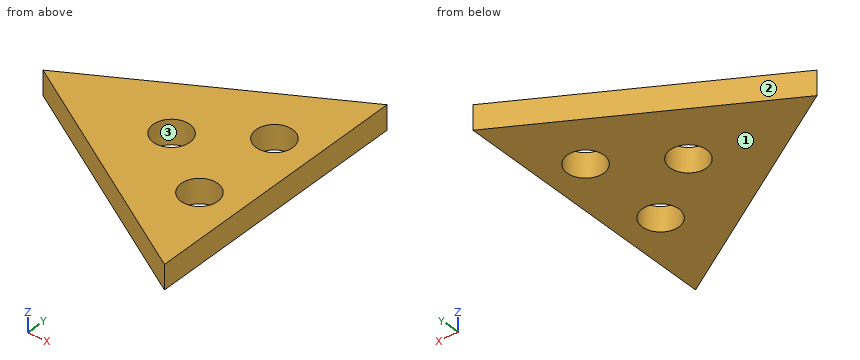
```python
from build123d import *

# Parameters (mm, degrees)
F0_R     = 1.5
F1_DEPTH = 2


with BuildPart() as f1:
    # F0 (on Top) → F1 (new body)
    with BuildSketch(Plane.XY):
        Polygon((9.526279, 11), (-9.526279, 0), (9.526279, -11), (9.526279, -10), (9.526279, 10), align=None)
        with Locations((6.350847, -3.708273)):
            Circle(F0_R, mode=Mode.SUBTRACT)
        with Locations((1, 0)):
            Circle(F0_R, mode=Mode.SUBTRACT)
        with Locations((6.350847, 3.708273)):
            Circle(F0_R, mode=Mode.SUBTRACT)
    extrude(amount=F1_DEPTH)


solid = f1.part
```
Geometry check sheet. Reference: the model listing, model coordinates, mm. Face numbers are marked on the shaded views. Coordinates: 2 decimals unless noted, no trailing zeros. Write each loop counter-clockwise with the first axis right and the second up, starting at its lowest first coordinate (ties: lowest second). Pieces come first, ordered by that corner, then holes. Notation, with made-up numbers: M 10.25,-11 L 30.25,-11 A14 cw 30.25,1 Z; hole C 56.25,-5.5 d7. An arc over 180 degrees is marked long. One line per item, written item: value. Start each with the question number.
(1) Scan lines: line 1 along Y through (x, z) = (7.25, 0.9); line 2 along Y through (x, z) = (5.5, 1.2); line 3 along X through (y, z) = (4, 1.65). Record each from-to range of solid material in increasing order. Write a range as [from, to].
(2) Release check for a two-part mould opening along Y. For the marked faces 1, 2 and 3 record: released by +Y, released by -Y, zero draft, split by the parting line, or undercut.
(3) Sectioned sample at C-C, the plane z = 0.55. Enter the section's corners in (x, y).
(4) Sectioned sample at A-A, the plane x = 1. Enter the section's corners in (y, z).
(5) Sectioned sample at D-D, the plane x = -7.75. Enter the section's corners in (y, z).
(6) Sectioned sample at B-B, the plane y = -0.5. Enter the section's corners in (x, z).
(7) Depth check by flat-ended pin: pin 1 (3.5 mm diameter, centred on x = 1, y = 0, fed in from +Z); pin 2 (2.5 mm diameter, centred on x = 6.35, y = -3.71, fed in from -Z); pin 3 (1 mm diameter, centred on x = 2.5, z = 2, fed in from +Y). Enter the tip coordinate at first touch or a pass-through.
Filled sheet:
1. line 1: [-9.69, -4.91], [-2.51, 2.51], [4.91, 9.69]
1. line 2: [-8.68, -4.94], [-2.47, 2.47], [4.94, 8.68]
1. line 3: [-2.6, 4.88], [7.82, 9.53]
2. face 1: zero draft
2. face 2: released by +Y
2. face 3: undercut
3. outline: M -9.53,0 L 9.53,-11 L 9.53,11 Z; hole C 1,0 d3; hole C 6.35,-3.71 d3; hole C 6.35,3.71 d3
4. outline: M -6.08,0 L -1.5,0 L -1.5,2 L -6.08,2 Z; M 1.5,0 L 6.08,0 L 6.08,2 L 1.5,2 Z
5. outline: M -1.03,0 L 1.03,0 L 1.03,2 L -1.03,2 Z
6. outline: M -8.66,0 L -0.41,0 L -0.41,2 L -8.66,2 Z; M 2.41,0 L 9.53,0 L 9.53,2 L 2.41,2 Z
7. pin 1: z = 2
7. pin 2: through
7. pin 3: y = 7.23
